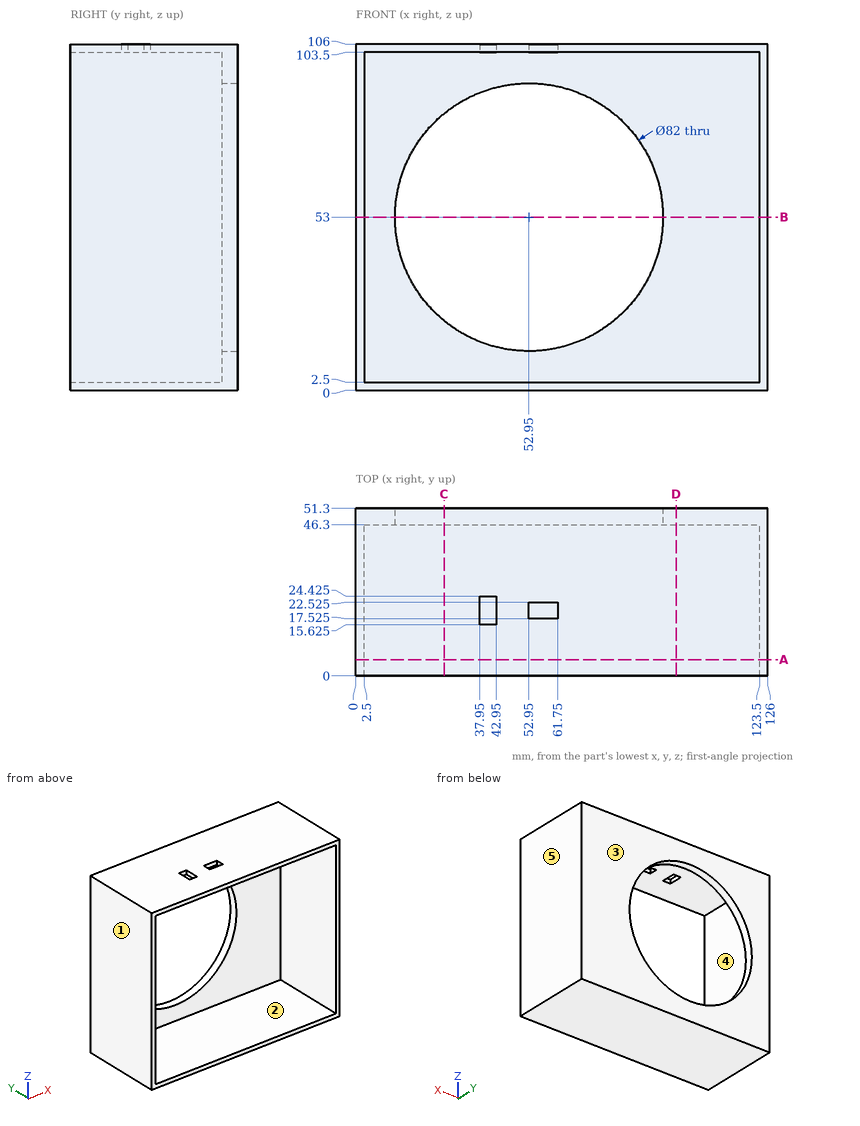
Input: dimensioned drawing with shaded views. Units: mm. Origin: part minimum x, y, z. A direction names the side the tool comes from. Coordinates: 2 decimals unless noted, no trailing zeros. Loops run counter-clockwise (first coordinate to the right, second up) from the corner with the lowest first, then second, coordinate; pieces in that order, holes last. Notation, with made-up numbers: (45.5, -6.75) -> (75.5, -6.75) arc R13 ccw to (75.5, 17.25) -> close; hole circle Ø6 at (74, -21.75). An arc over 180 degrees is marked (long way). Use a Markdown table: item, result. Add a question column.
(1) Section query D-D, the plane x = 98. Return loops of the section in (y, z), plus the area to 4 significant figures.
(2) Section query B-B, the plane z = 53. Return loops of the section in (x, y), plus the area to 4 significant figures.
(3) Section query A-A, the plane y = 5. Return loops of the section in (x, z), plus the area to 4 significant figures.
(4) Line query: line 1 along X through (y, z) = (49.7, 53); line 2 along X through (y, z) = (13.5, 15); line 3 along Z through (x, y) = (52.95, 50.15). Output: solid intervals per line, ascending.
(5) Section query C-C, the plane x = 27. Return loops of the section in (y, z), plus the area to 3 significant figures.
(6) Mould query, pull axis X, two halves, no side actions, for the marked faces 1, 2 and 3. Classes: pulls with the +X half, pulls with the -X half, needs draft (parallel to the pull), parting line crosses it, or undercut.
(7) Access query for the marked faces 4 and 5. Directions: +Z, -Z, +X, -X, +Y, -Y. A direction counts if a zero-diameter tool reaches every point of the face in a straight line with its end or side. Return the directions, or none.
(8) Pin query (flat end, axial travel): pin 1 Ø4 at (x, z) = (98, 53.5) entering from -Y. Return the tip coordinate at first contact, or that it passes through.
Answer:
| question | item | result |
|---|---|---|
| 1 | outline | (0, 0) -> (51.3, 0) -> (51.3, 106) -> (0, 106) -> (0, 103.5) -> (46.3, 103.5) -> (46.3, 2.5) -> (0, 2.5) -> close |
| 1 | area | 761.5 mm^2 |
| 2 | outline | (0, 0) -> (2.5, 0) -> (2.5, 46.3) -> (11.95, 46.3) -> (11.95, 51.3) -> (0, 51.3) -> close; (93.95, 46.3) -> (123.5, 46.3) -> (123.5, 0) -> (126, 0) -> (126, 51.3) -> (93.95, 51.3) -> close |
| 2 | area | 451.5 mm^2 |
| 3 | outline | (0, 0) -> (126, 0) -> (126, 106) -> (0, 106) -> close; hole (2.5, 2.5) -> (123.5, 2.5) -> (123.5, 103.5) -> (2.5, 103.5) -> close |
| 3 | area | 1,135 mm^2 |
| 4 | line 1 | x = 0 to 11.95, 93.95 to 126 |
| 4 | line 2 | x = 0 to 2.5, 123.5 to 126 |
| 4 | line 3 | z = 0 to 12, 94 to 106 |
| 5 | outline | (0, 0) -> (51.3, 0) -> (51.3, 21.26) -> (46.3, 21.26) -> (46.3, 2.5) -> (0, 2.5) -> close; (0, 103.5) -> (46.3, 103.5) -> (46.3, 84.74) -> (51.3, 84.74) -> (51.3, 106) -> (0, 106) -> close |
| 5 | area | 444 mm^2 |
| 6 | face 1 | pulls with the -X half |
| 6 | face 2 | undercut |
| 6 | face 3 | needs draft |
| 7 | face 4 | -Y |
| 7 | face 5 | +Z, -Z, +X, +Y, -Y |
| 8 | pin 1 | stops at y = 46.3 |
